from build123d import *

# Parameters (mm, degrees)
BOSS_EXTRUDE1_DEPTH = 12
SKETCH2_W           = 12
SKETCH2_H           = 300
CUT_EXTRUDE1_DEPTH  = 6


with BuildPart() as part:
    # Sketch1 → Boss-Extrude1 (new body)
    with BuildSketch(Plane.XY):
        with BuildLine():
            Line((45.562175866, 543.226317211), (245.677247379, 302.584656473))
            Line((245.677247379, 302.584656473), (266.942237958, 277.013155986))
            ThreePointArc((266.942237958, 277.013155986), (270.373567716, 271.024119998), (271.564632115, 264.225300867))
            Line((271.564632115, 264.225300867), (271.564632115, 250.438462092))
            Line((271.564632115, 250.438462092), (289.564632115, 250.438462092))
            Line((289.564632115, 250.438462092), (289.564632115, -49.561537908))
            Line((289.564632115, -49.561537908), (-310.435367885, -49.561537908))
            Line((-310.435367885, -49.561537908), (-310.435367885, 550.438462092))
            Line((-310.435367885, 550.438462092), (30.184570023, 550.438462092))
            ThreePointArc((30.184570023, 550.438462092), (38.677004822, 548.545879113), (45.562175866, 543.226317211))
        make_face()
        with BuildLine():
            Line((-1.540507591, -4.561537908), (-1.540507591, 505.438462092))
            ThreePointArc((-1.540507591, 505.438462092), (11.660673278, 524.247397693), (33.837098252, 518.226317211))
            Line((33.837098252, 518.226317211), (241.942237958, 267.976468219))
            ThreePointArc((241.942237958, 267.976468219), (245.373567716, 261.98743223), (246.564632115, 255.1886131))
            Line((246.564632115, 255.1886131), (246.564632115, -4.561537908))
            ThreePointArc((246.564632115, -4.561537908), (240.706767739, -18.703673532), (226.564632115, -24.561537908))
            Line((226.564632115, -24.561537908), (18.459492409, -24.561537908))
            ThreePointArc((18.459492409, -24.561537908), (4.317356785, -18.703673532), (-1.540507591, -4.561537908))
        make_face(mode=Mode.SUBTRACT)
    extrude(amount=-BOSS_EXTRUDE1_DEPTH)

    # Sketch2 → Cut-Extrude1 (cut)
    with BuildSketch(Plane(origin=(0, 0, -12), x_dir=(-1, 0, 0), z_dir=(0, 0, -1))):
        with Locations((-277.564632115, 100.438462092)):
            Rectangle(SKETCH2_W, SKETCH2_H)
    extrude(amount=-CUT_EXTRUDE1_DEPTH, mode=Mode.SUBTRACT)


solid = part.part
The model under review builds one solid part; all positions refer to its coordinate system, in mm. A direction names the side the tool comes from. Coordinates: 2 decimals unless noted, no trailing zeros. Write each loop counter-clockwise with the first axis right and the second up, starting at its lowest first coordinate (ties: lowest second). Pieces come first, ordered by that corner, then holes. Notation, with made-up numbers: (33, -12.75) - (68, -12.75) arc R15 ccw to (68, -6.75) - close; hole circle Ø10 at (67, 77.25). An arc over 180 degrees is marked (long way). Answer as a JSON object with one key per item and string values. Group by question number.
1. Add section D-D (x = 212.5). Give the boundary of the cut face in (y, z).
2. Machinability: for faces 3 (the face through (-73, 255, 0)), 4 (the face through (136.433, 394.853, -5.916)), which of the approach directions +Z, -Z, +X, -X, +Y, -Y give a long, thin tool a straight path to every point of the face, cutting with its end or side? Answer none if there is none.
3. Mouldability with a two-part tool opening along X and no side actions: class faces 1 (the face through (-145, 255, -12)), 2 (the face through (4.474, -18.858, -5.916)) as pulls with the +X half, pulls with the -X half, needs draft (parallel to the pull), parting line crosses it, or undercut.
4. Add section A-A (z = -4). Give the boundary of the cut face in (x, y).
5. To check wall thickness, follow probe 1 along X at (y, z) = (176, -11.25); probe 2 along X at (y, z) = (38.5, -2.25); probe 3 along Y at (x, z) = (244.5, -7.25). State the ranges of each line that lie inside material, in increasing order.
6. Add section B-B (y = 102). Give the boundary of the cut face in (x, z).
7. Add section C-C (x = 6). Give the boundary of the cut face in (y, z).
8. Clearance check with flat-ended pins moving along their axes: pin 1 Ø3.5 at (y, z) = (276, -4) entering from +X; pin 2 Ø3.5 at (x, y) = (280, 81.5) entering from -Z. State where each tip first meets the part, or that it passes through.
Findings:
{
 "1": {"outline": "(-49.56, -12) - (-24.56, -12) - (-24.56, 0) - (-49.56, 0) - close; (303.38, -12) - (342.48, -12) - (342.48, 0) - (303.38, 0) - close"},
 "2": {"face 3": "+Z, +X, -X, +Y, -Y", "face 4": "+Z, -Z"},
 "3": {"face 1": "needs draft", "face 2": "undercut"},
 "4": {"outline": "(-310.44, -49.56) - (289.56, -49.56) - (289.56, 250.44) - (271.56, 250.44) - (271.56, 264.23) arc R20 ccw to (266.94, 277.01) - (45.56, 543.23) arc R20 ccw to (30.18, 550.44) - (-310.44, 550.44) - close; hole (-1.54, -4.56) arc R20 ccw to (18.46, -24.56) - (226.56, -24.56) arc R20 ccw to (246.56, -4.56) - (246.56, 255.19) arc R20 ccw to (241.94, 267.98) - (33.84, 518.23) arc R20 ccw to (-1.54, 505.44) - close"},
 "5": {"probe 1": "-310.44 to -1.54, 246.56 to 271.56, 283.56 to 289.56", "probe 2": "-310.44 to -1.54, 246.56 to 289.56", "probe 3": "-49.56 to -13.41, 264.04 to 304"},
 "6": {"outline": "(-310.44, -12) - (-1.54, -12) - (-1.54, 0) - (-310.44, 0) - close; (246.56, -12) - (271.56, -12) - (271.56, -6) - (283.56, -6) - (283.56, -12) - (289.56, -12) - (289.56, 0) - (246.56, 0) - close"},
 "7": {"outline": "(-49.56, -12) - (-20.21, -12) - (-20.21, 0) - (-49.56, 0) - close; (521.08, -12) - (550.44, -12) - (550.44, 0) - (521.08, 0) - close"},
 "8": {"pin 1": "x = 268.87", "pin 2": "z = -6"}
}
